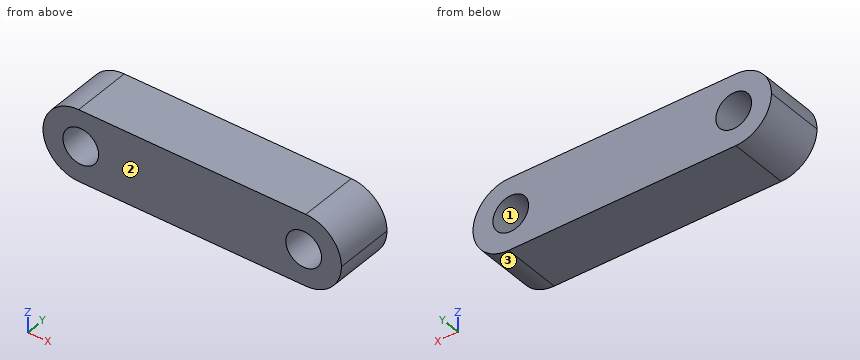
from build123d import *

# Parameters (mm, degrees)
SKETCH1_W           = 50.2
SKETCH1_H           = 12
SKETCH1_R           = 3
BOSS_EXTRUDE1_DEPTH = 10
FILLET1_R           = 6


with BuildPart() as part:
    # Sketch1 → Boss-Extrude1 (new body)
    with BuildSketch(Plane(origin=(0, 0, 0), x_dir=(1, 0, 0), z_dir=(0, 1, 0))):
        Rectangle(SKETCH1_W, SKETCH1_H)
        with Locations(Location((18.75, 0, 0), (0, 0, 270))):
            Circle(SKETCH1_R, mode=Mode.SUBTRACT)
        with Locations(Location((-18.75, 0, 0), (0, 0, 270))):
            Circle(SKETCH1_R, mode=Mode.SUBTRACT)
    extrude(amount=BOSS_EXTRUDE1_DEPTH)

    # Fillet1
    fillet1_edges = [part.edges().sort_by_distance(p)[0] for p in [
        (25.1, 5, -6),
        (25.1, 5, 6),
        (-25.1, 5, -6),
        (-25.1, 5, 6),
    ]]
    fillet(fillet1_edges, radius=FILLET1_R - 0.0001)  # a hair under: the kernel refuses the full size


solid = part.part
The model under review builds one solid part; all positions refer to its coordinate system, in mm. Face numbers are marked on the shaded views. Round coordinates to 2 decimals unless told otherwise and drop trailing zeros. Order: outer loops, then holes, each group sorted by start corner. A loop starts at its lowest first (then second) coordinate and runs counter-clockwise, first axis right, second up. Notation, with made-up numbers: (-29, 65) -> (17, 65) arc R22 ccw to (17, 86) -> close; hole circle Ø4 at (65.25, 70). An arc over 180 degrees is marked (long way). Return JSON: item names as keys, results as strings.
1. The part is to be moulded in two halves that separate along X. For the marked faces 1, 2 and 3, say which applies: +X half, -X half, draft (parallel to the pull), parting line (faces both ways), or undercut.
Answer block:
{"face 1": "undercut", "face 2": "draft", "face 3": "+X half"}
2. For L1, parallel to X at y = 6.5, z = 0; L2, parallel to X at y = 5.5, z = -1.75; L3, parallel to Z at x = 21, y = 2, list the stretches that pass through material, from the lowest coordinate up. Write a range as [from, to].
Answer block:
{"L1": "x = [-25.1, -21.75], [-15.75, 15.75], [21.75, 25.1]", "L2": "x = [-24.84, -21.19], [-16.31, 16.31], [21.19, 24.84]", "L3": "z = [-5.69, -1.98], [1.98, 5.69]"}
3. Take a section at C-C (x = 17.5). Write out the cut boundary in (y, z).
Answer block:
{"outline": "(0, -6) -> (10, -6) -> (10, -2.73) -> (0, -2.73) -> close; (0, 2.73) -> (10, 2.73) -> (10, 6) -> (0, 6) -> close"}
4. Take a section at A-A (y = 6.75). State how many separate pieces and enclosed holes the cut face has, then the cut area to 3 significant figures.
Answer block:
{"separate pieces": "1", "enclosed holes": "2", "area": "515 mm²"}
5. Take a section at D-D (z = 2). Write out the cut boundary in (x, y), then the cut area to 3 significant figures.
Answer block:
{"outline": "(-24.76, 0) -> (-20.99, 0) -> (-20.99, 10) -> (-24.76, 10) -> close; (-16.51, 0) -> (16.51, 0) -> (16.51, 10) -> (-16.51, 10) -> close; (20.99, 0) -> (24.76, 0) -> (24.76, 10) -> (20.99, 10) -> close", "area": "406 mm²"}
6. Take a section at B-B (z = -1.25). Write out the cut boundary in (x, y).
Answer block:
{"outline": "(-24.97, 0) -> (-21.48, 0) -> (-21.48, 10) -> (-24.97, 10) -> close; (-16.02, 0) -> (16.02, 0) -> (16.02, 10) -> (-16.02, 10) -> close; (21.48, 0) -> (24.97, 0) -> (24.97, 10) -> (21.48, 10) -> close"}
